Autodesk Inventor part; units mm, degrees
ref_plane "Work Plane2" through (2.8, 0, 0) normal (0, 1, 0) x (1, 0, 0)
ref_plane "YZ Plane" through (0, 0, 0) normal (1, 0, 0) x (0, 1, 0)
ref_plane "XZ Plane" through (0, 0, 0) normal (0, 1, 0) x (-1, 0, 0)
sketch "Sketch1" plane through (0, 0, 0) normal (0, 0, 1) x (1, 0, 0)
  line L0 (3.5, 0) -> (25, 0)
  line L1 (25, 0) -> (25, 3.15)
  line L2 (25, 3.15) -> (3.15, 3.15)
  line L3 (0.65, 5.65) -> (0, 5.65)
  line L4 (-5, 0) -> (30, 0)
  line L5 (0, -1.13) -> (0, 6.78)
  line L6 (0, 3.4) -> (2.3026, 2.252)
  line L7 (2.3026, 2.252) -> (3.5, 0)
  line L8 (3.15, 3.15) -> (0.65, 5.65)
  line L9 (0, 5.65) -> (0, 3.4)
  dimension "d2" = 6.3
  dimension "d3" = 11.3
  dimension "d4" = 3.5
  dimension "d5" = 6.8
  dimension "d6" = 26.5
  dimension "d7" = 62
  dimension "d13" = 45
  dimension "d14" = 3.15
  dimension "d15" = 25
revolve "Body" add sketch "Sketch1" angle 360 about axis through (3.5, 0, 0) along (1, 0, 0) contours L7 L6 L5 L3 L8 L2 L1 L0
sketch "Sketch2" plane through (0, 0, 0) normal (-1, 0, 0) x (0, 0, 1)
  line L0 (0, -7.91) -> (0, 7.91)
  line L1 (-7.91, 0) -> (7.91, 0)
  line L2 (0, 3.4) -> (0, 0) construction
  line L3 (0, 0) -> (3.4, 0) construction
  arc A0 (1.02, 0) -> (0, 1.02) centre (0, 0) ccw construction
  line L4 (0, 0) -> (3.9952, 3.9952) construction
  arc A1 (1.19, 0) -> (0, 1.19) centre (0, 0) ccw construction
  line L5 (0.395, 3.377) -> (0.5735, 1.0427)
  line L6 (3.377, 0.395) -> (1.0427, 0.5735)
  arc A2 (0.5735, 1.0427) -> (1.0427, 0.5735) centre (1.0815, 1.0815) ccw
  arc A3 (3.4, 0) -> (3.377, 0.395) centre (0, 0) ccw
  arc A4 (0.395, 3.377) -> (0, 3.4) centre (0, 0) ccw
  arc A5 (3.377, 0.395) -> (0.395, 3.377) centre (0, 0) ccw
  line L7 (0.395, -3.377) -> (0.5735, -1.0427)
  line L8 (3.377, -0.395) -> (1.0427, -0.5735)
  arc A6 (1.0427, -0.5735) -> (0.5735, -1.0427) centre (1.0815, -1.0815) ccw
  arc A7 (3.377, -0.395) -> (3.4, 0) centre (0, 0) ccw
  arc A8 (0, -3.4) -> (0.395, -3.377) centre (0, 0) ccw
  arc A9 (0.395, -3.377) -> (3.377, -0.395) centre (0, 0) ccw
  line L9 (-0.395, 3.377) -> (-0.5735, 1.0427)
  line L10 (-3.377, 0.395) -> (-1.0427, 0.5735)
  arc A10 (-1.0427, 0.5735) -> (-0.5735, 1.0427) centre (-1.0815, 1.0815) ccw
  arc A11 (-3.377, 0.395) -> (-3.4, 0) centre (0, 0) ccw
  arc A12 (0, 3.4) -> (-0.395, 3.377) centre (0, 0) ccw
  arc A13 (-0.395, 3.377) -> (-3.377, 0.395) centre (0, 0) ccw
  arc A14 (-3.377, -0.395) -> (-0.395, -3.377) centre (0, 0) ccw
  arc A15 (-0.395, -3.377) -> (0, -3.4) centre (0, 0) ccw
  arc A16 (-3.4, 0) -> (-3.377, -0.395) centre (0, 0) ccw
  line L11 (-3.377, -0.395) -> (-1.0427, -0.5735)
  arc A17 (-0.5735, -1.0427) -> (-1.0427, -0.5735) centre (-1.0815, -1.0815) ccw
  line L12 (-0.395, -3.377) -> (-0.5735, -1.0427)
  circle A18 centre (0, 0) radius 5.65
  circle A19 centre (0, 0) radius 3.4
  dimension "d18" = 45
  dimension "d19" = 2.04
  dimension "d20" = 2.38
  dimension "d21" = 6.8
  dimension "d22" = 0.395
extrude "Slot" add sketch "Sketch2" against normal up to next draft 1 contours L7 A6 L8 A9 | A14 L11 A17 L12 | A13 L9 A10 L10 | L6 A2 L5 A5
fillet "Fillet1" radius 0.158 4 edges at (0, 3.4, 0) (0, 0, 3.4) (0, -3.4, 0) (0, 0, -3.4)
thread "Thread"
chamfer "Chamfer1" distance 0.875 distance2 3.6 1 edges at (25, -3.15, 0) measured on face at (25, 1.1633, 0.933)
ref_plane "Work Plane2" through (2.8, 0, 0) normal (0, 1, 0) x (1, 0, 0)
equation "\"d2\" = NND"
equation "\"d3\" = KOD"
equation "\"d4\" = STI"
equation "\"d5\" = SDM"
equation "\"d13\" = 0.5 * SEWI"
equation "\"d14\" = KOH"
equation "\"d15\" = NLG"
equation "\"d19\" = 0.3 * SDM"
equation "\"d20\" = 0.35 * SDM"
equation "\"d21\" = SDM"
equation "\"d22\" = 0.5 * SBR"
equation "\"d45\" = STI"
equation "\"d25\" = 0.2 * SBR"
equation "\"d9\" = GEL"
equation "\"d11\" = -0.5 * GD2 + 0.5 * NND"
equation "\"d12\" = SPTZ"
equation "\"NND\" = 6.3"
equation "\"NLG\" = 25"
equation "\"GEL\" = 21.85"
equation "\"KOD\" = 11.3"
equation "\"KOH\" = 3.15"
equation "\"SDM\" = 6.8"
equation "\"STI\" = 3.5"
equation "\"SBR\" = 0.79"
equation "\"SPTZ\" = 3.6"
equation "\"GD2\" = 4.55"
equation "\"SEWI\" = 90deg"
equation "\"d0\" = NLG"
equation "\"d1\" = KOH"
equation "\"d17\" = SDM"
equation "\"EPV\" = 6.3"
equation "\"THREADDIA\" = 6.3"
equation "\"TOA\" = 30deg"
equation "\"PTC\" = 1.8"
equation "\"GD1\" = 4.88"
properties part number "ISO 7050 - ST6,3 x 25 - F - H" material "Steel"
Model file for the job. Use its own axes, mm. A direction names the side the tool comes from. Round coordinates to 2 decimals unless told otherwise and drop trailing zeros. Loops run counter-clockwise (first coordinate to the right, second up) from the corner with the lowest first, then second, coordinate; pieces in that order, holes last.
1. Drop flat-ended pins along their axis: P1, Ø6, axis at x = 4.5, z = -2.5, coming from the -Y side; P2, Ø5, axis at y = -2.5, z = 0, coming from the +X side; P3, Ø5, axis at x = 19.5, z = -1, coming from the +Y side; P4, Ø2, axis at x = 13.5, z = -3.5, coming from the +Y side. Give the stop position or say it passes through.
Check values:
P1: stops at y = -4.38
P2: stops at x = 25
P3: stops at y = 3.15
P4: stops at y = 1.92
2. Tool access for faces 4 (the cylindrical face through (12.147, -2.5, 1.917)), 5 (the flat face through (25, 0, 0)), 6 (the conical face through (1.4, -2.7, 0)): list every direction of +Z, -Z, +X, -X, +Y, -Y with a clear straight run to the whole face (end or side of a thin tool).
Check values:
face 4: +X
face 5: +Z, -Z, +X, +Y, -Y
face 6: -X
3. Band-saw the part on A-A, the plane x = 16.25. List the corners of the cut face in (y, z), and give its area (3 significant figures).
Check values:
outline: circle Ø6.3 at (0, 0)
area: 31.2 mm2
4. Wall check: probe 1 along Z at (x, y) = (14.75, 2.25); probe 2 along Y at (x, z) = (18, 1.25); probe 3 along Z at (x, y) = (18, -1.5). Give the ranges that are in metal, low to high.
Check values:
probe 1: z = -2.2 to 2.2
probe 2: y = -2.89 to 2.89
probe 3: z = -2.77 to 2.77
5. Mould opens along Z. For faces 1 (the cylindrical face through (0.32, 5.39, -1.7)), 2 (the conical face through (1.4, 2.7, 0)), 3 (the flat face through (0, 1, -1)) say: +Z half, -Z half, draft (parallel to the pull), parting line (faces both ways), or undercut.
Check values:
face 1: parting line
face 2: undercut
face 3: draft
